Geometry check sheet. Reference: drawing and pictorial views, mm from the part's lowest x, y, z. Round coordinates to 2 decimals unless told otherwise and drop trailing zeros. Order: outer loops, then holes, each group sorted by start corner. A loop starts at its lowest first (then second) coordinate and runs counter-clockwise, first axis right, second up.
(1) Release check for a two-part mould opening along Y. For the marked faces 1, 2 and 3 record: +Y half, -Y half, draft (parallel to the pull), parting line (faces both ways), or undercut.
(2) Sectioned sample at C-C (z = 5.25). Record the boundary of the cut face in (x, y) (1 decimal).
(3) Material ranges on line 1 along Y through (x, z) = (2.3, 4.5) (1 decimal); line 2 along X through (y, z) = (3.2, 2) (1 decimal); line 3 along Z through (x, y) = (2.85, 0.95), recorded low to high.
(4) Go/stop test with flat-tipped pins: pin 1 (1.5 mm diameter, centred on y = 3.5, z = 5, fed in from +X); pin 2 (1.4 mm diameter, centred on x = 3, z = 0.5, fed in from +Y); pin 3 (1.5 mm diameter, centred on x = 2, y = 3.5, fed in from -Z) (1 decimal). Record where each tip stops, or that it passes through.
(5) Sectioned sample at B-B (x = 3.25). Record the boundary of the cut face in (y, z).
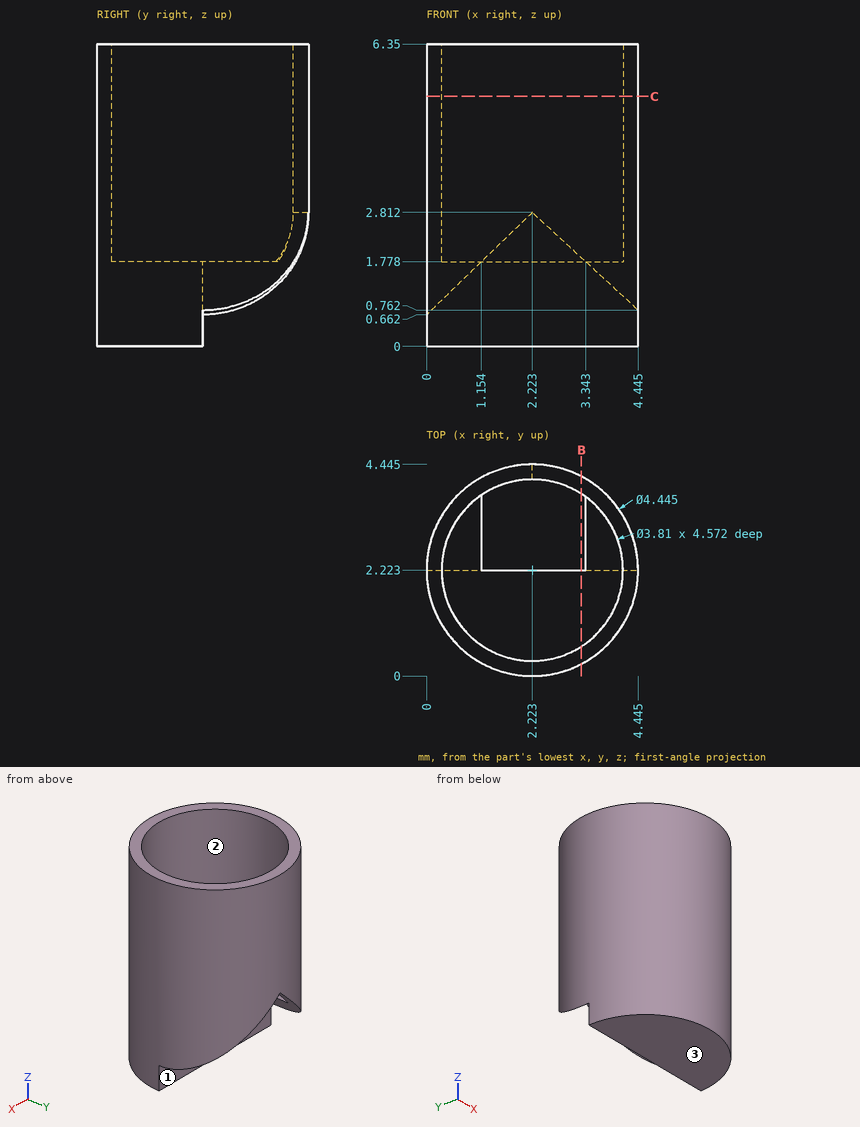
Answer below:
1. face 1: +Y half
1. face 2: undercut
1. face 3: draft
2. outline: circle Ø4.4 at (2.2, 2.2); hole circle Ø3.8 at (2.2, 2.2)
3. line 1: y = 0 to 0.3, 4.1 to 4.4
3. line 2: x = 0.2 to 0.6, 3.9 to 4.2
3. line 3: z = 0 to 1.78
4. pin 1: stops at x = 4.38
4. pin 2: stops at y = 2.22
4. pin 3: stops at z = 2
5. outline: (0.25, 0) - (2.22, 0) - (2.22, 1.78) - (0.62, 1.78) - (0.62, 6.35) - (0.25, 6.35) - close; (3.83, 1.86) - (4.19, 1.86) - (4.19, 6.35) - (3.83, 6.35) - close
